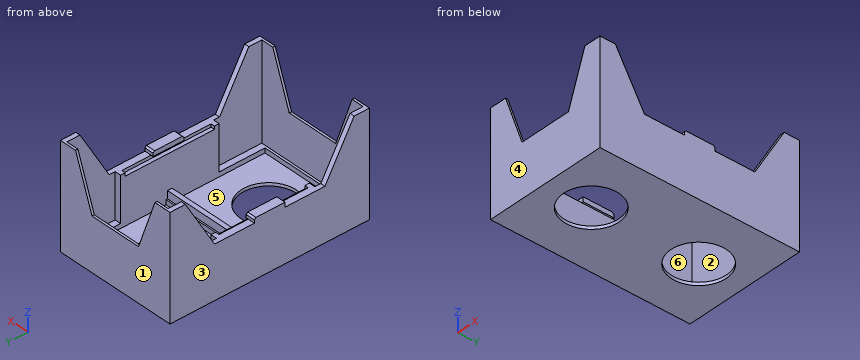
```python
from build123d import *

# Parameters (mm, degrees)
SKETCH1_W                    = 130
SKETCH1_H                    = 80
SKETCH1_R                    = 18
BOSS_EXTRUDE1_DEPTH          = 2
SKETCH2_W                    = 7
SKETCH2_H                    = 130
BOSS_EXTRUDE2_DEPTH          = 30
BOSS_EXTRUDE3_DEPTH          = 35
SKETCH5_W                    = 150
SKETCH5_H                    = 110
CUT_EXTRUDE1_DEPTH           = 33
CUT_EXTRUDE1_DRAFT           = -30
SKETCH6_W                    = 6
SKETCH6_H                    = 20
BOSS_EXTRUDE4_DEPTH          = 3
CHAMFER1_SIZE                = 1
SKETCH7_W                    = 80
SKETCH7_H                    = 5
SKETCH7_H_2                  = 3
BOSS_EXTRUDE5_DEPTH          = 3
SKETCH9_W                    = 74
SKETCH9_H                    = 32.9
CUT_EXTRUDE2_DEPTH           = 99.33107342
SKETCH10_W                   = 72.40522931
SKETCH10_H                   = 3
BOSS_EXTRUDE6_DEPTH          = 5
SKETCH11_W                   = 80
SKETCH11_H                   = 1.5
BOSS_EXTRUDE7_DEPTH          = 62
SKETCH12_W                   = 58
SKETCH12_H                   = 28.83651326
CUT_EXTRUDE3_DEPTH           = 33
CUT_EXTRUDE3_DRAFT           = -20
CUT_EXTRUDE3_PROFILE_2_DEPTH = 33
CUT_EXTRUDE3_PROFILE_2_DRAFT = -20


with BuildPart() as part:
    # Sketch1 → Boss-Extrude1 (new body)
    with BuildSketch(Plane(origin=(0, 0, 0), x_dir=(0, 1, 0), z_dir=(0, 0, 1))):
        Rectangle(SKETCH1_W, SKETCH1_H)
        with Locations(Location((-35, 0, 0), (0, 0, 270))):
            Circle(SKETCH1_R, mode=Mode.SUBTRACT)
        with Locations(Location((35, 0, 0), (0, 0, 90))):
            Circle(SKETCH1_R, mode=Mode.SUBTRACT)
    extrude(amount=BOSS_EXTRUDE1_DEPTH)

    # Sketch2 → Boss-Extrude2 (add)
    with BuildSketch(Plane.XY.offset(2)):
        with Locations((-36.5, 0)):
            Rectangle(SKETCH2_W, SKETCH2_H)
        with Locations((36.5, 0)):
            Rectangle(SKETCH2_W, SKETCH2_H)
    extrude(amount=BOSS_EXTRUDE2_DEPTH)

    # Sketch4 → Boss-Extrude3 (add)
    with BuildSketch(Plane.XY.offset(32)):
        Polygon((-33, 29.1), (-35.5, 29.1), (-35.5, -29.1), (-33, -29.1), (-33, -65), (-40, -65), (-40, 65), (-33, 65), align=None)
        Polygon((35.5, -29.1), (35.5, 29.1), (33, 29.1), (33, 65), (40, 65), (40, -65), (33, -65), (33, -29.1), align=None)
    extrude(amount=BOSS_EXTRUDE3_DEPTH)


with BuildPart() as cut_extrude1_tool:
    # Sketch5 → Cut-Extrude1 (with draft: the straight prism first)
    with BuildSketch(Plane.XY.offset(67)):
        Rectangle(SKETCH5_W, SKETCH5_H)
    extrude(amount=-CUT_EXTRUDE1_DEPTH)
    # Cut-Extrude1: the draft: its side faces are tilted about the plane it starts from
    cut_extrude1_sides = [cut_extrude1_tool.faces().sort_by_distance(p)[0] for p in [
        (0, -55, 50.5),
        (75, 0, 50.5),
        (0, 55, 50.5),
        (-75, 0, 50.5),
    ]]
    draft(cut_extrude1_sides, Plane.XY.offset(67), CUT_EXTRUDE1_DRAFT)


with BuildPart() as part_1:
    add(part.part)

    # Cut-Extrude1: cut by cut_extrude1_tool
    add(cut_extrude1_tool.part, mode=Mode.SUBTRACT)

    # Sketch6 → Boss-Extrude4 (add)
    with BuildSketch(Plane.XY.offset(34)):
        with Locations((37, 0)):
            Rectangle(SKETCH6_W, SKETCH6_H)
        with Locations((-37, 0)):
            Rectangle(SKETCH6_W, SKETCH6_H)
    extrude(amount=BOSS_EXTRUDE4_DEPTH)

    # Chamfer1
    chamfer1_edges = [part_1.edges().sort_by_distance(p)[0] for p in [
        (37, 10, 37),
        (37, -10, 37),
        (-37, 10, 37),
    ]]
    chamfer(chamfer1_edges, length=CHAMFER1_SIZE)

    # Sketch7 → Boss-Extrude5 (add)
    with BuildSketch(Plane.XY.offset(2)):
        Rectangle(SKETCH7_W, SKETCH7_H)
        with Locations((0, -63.5)):
            Rectangle(SKETCH7_W, SKETCH7_H_2)
        with Locations((0, 63.5)):
            Rectangle(SKETCH7_W, SKETCH7_H_2)
    extrude(amount=BOSS_EXTRUDE5_DEPTH)

    # Sketch9 → Cut-Extrude2 (cut, through all)
    with BuildSketch(Plane.XY.offset(5)):
        with Locations((0, 48.55)):
            Rectangle(SKETCH9_W, SKETCH9_H)
        with Locations((0, -48.55)):
            Rectangle(SKETCH9_W, SKETCH9_H)
    extrude(amount=CUT_EXTRUDE2_DEPTH, mode=Mode.SUBTRACT)

    # Sketch10 → Boss-Extrude6 (add)
    with BuildSketch(Plane.XY.offset(5)):
        Rectangle(SKETCH10_W, SKETCH10_H)
    extrude(amount=BOSS_EXTRUDE6_DEPTH)

    # Sketch11 → Boss-Extrude7 (add)
    with BuildSketch(Plane.XY.offset(5)):
        with Locations((0, 64.25)):
            Rectangle(SKETCH11_W, SKETCH11_H)
        with Locations((0, -64.25)):
            Rectangle(SKETCH11_W, SKETCH11_H)
    extrude(amount=BOSS_EXTRUDE7_DEPTH)


with BuildPart() as cut_extrude3_tool:
    # Sketch12 → Cut-Extrude3 (with draft: the straight prism first)
    with BuildSketch(Plane.XY.offset(67)):
        with Locations((0, 63.5)):
            Rectangle(SKETCH12_W, SKETCH12_H)
    extrude(amount=-CUT_EXTRUDE3_DEPTH)
    # Cut-Extrude3: the draft: its side faces are tilted about the plane it starts from
    cut_extrude3_sides = [cut_extrude3_tool.faces().sort_by_distance(p)[0] for p in [
        (0, 49.08174337, 50.5),
        (29, 63.5, 50.5),
        (0, 77.91825663, 50.5),
        (-29, 63.5, 50.5),
    ]]
    draft(cut_extrude3_sides, Plane.XY.offset(67), CUT_EXTRUDE3_DRAFT)


with BuildPart() as part_2:
    add(part_1.part)

    # Cut-Extrude3: cut by cut_extrude3_tool
    add(cut_extrude3_tool.part, mode=Mode.SUBTRACT)


with BuildPart() as cut_extrude3_profile_2_tool:
    # Sketch12 → Cut-Extrude3 profile 2 (with draft: the straight prism first)
    with BuildSketch(Plane.XY.offset(67)):
        with Locations((0, -63.5)):
            Rectangle(SKETCH12_W, SKETCH12_H)
    extrude(amount=-CUT_EXTRUDE3_PROFILE_2_DEPTH)
    # Cut-Extrude3 profile 2: the draft: its side faces are tilted about the plane it starts from
    cut_extrude3_profile_2_sides = [cut_extrude3_profile_2_tool.faces().sort_by_distance(p)[0] for p in [
        (-29, -63.5, 50.5),
        (0, -77.91825663, 50.5),
        (29, -63.5, 50.5),
        (0, -49.08174337, 50.5),
    ]]
    draft(cut_extrude3_profile_2_sides, Plane.XY.offset(67), CUT_EXTRUDE3_PROFILE_2_DRAFT)


with BuildPart() as part_3:
    add(part_2.part)

    # Cut-Extrude3 profile 2: cut by cut_extrude3_profile_2_tool
    add(cut_extrude3_profile_2_tool.part, mode=Mode.SUBTRACT)


solid = part_3.part
```
Geometry: final body of the model. Coordinates: model frame, mm. Face numbers are marked on the shaded views. A direction names the side the tool comes from. Give positions to 0.01 mm unless a question says otherwise; leave off trailing zeros. Loops run counter-clockwise (first coordinate to the right, second up) from the corner with the lowest first, then second, coordinate; pieces in that order, holes last. Notation, with made-up numbers: (-5, 83.5) - (14, 83.5) arc R22 ccw to (14, 122.5) - close; hole circle Ø9 at (60.5, -35). An arc over 180 degrees is marked (long way). Answer as CSV lines item,"result". Start each with the question number.
(1) Section query D-D (y = -56.5). Output: boundary loops of the cut face in (x, z).
(2) Section query B-B (z = 55.5). Output: boundary loops of the cut face in (x, y), and give its area (3 significant figures).
(3) Reachability of the marked faces 1 and 2 from +Z, -Z, +X, -X, +Y, -Y: full face, straight path, thin tool, end or side. Return the list, or none.
(4) Mould query, pull axis X, two halves, no side actions, for the marked faces 3, 4, 5 and 6. Classes: +X half, -X half, draft (parallel to the pull), parting line (faces both ways), or undercut.
(5) Section query A-A (z = 25). Output: boundary loops of the cut face in (x, y).
(6) Ray query, line 1 along Y through (x, z) = (0, 0.55); line 2 along X through (y, z) = (-57, 55); line 3 along X through (y, z) = (-14, 16.5). Return the intervals inside material, ascending. Write a range as [from, to].
(7) Section query C-C (x = 11). Output: boundary loops of the cut face in (y, z).
(8) Pin query (flat end, axial travel): P1, Ø3, axis at x = -34, y = 9.5, coming from the +Z side; P2, Ø0.5, axis at x = -9, y = -2, coming from the +Z side; P3, Ø3.5, axis at x = -35.5, y = -26.5, coming from the +Z side; P4, Ø10, axis at y = 19.5, z = 43, coming from the +X side. Return the tip coordinate at first contact, or that it passes through.
Worked answers:
1,outline,"(-40, 0) - (40, 0) - (40, 67) - (37, 67) - (37, 5) - (33, 5) - (33, 2) - (-33, 2) - (-33, 5) - (-37, 5) - (-37, 67) - (-40, 67) - close"
2,outline,"(-40, -65) - (-24.81, -65) - (-24.81, -63.5) - (-37, -63.5) - (-37, -48.36) - (-40, -48.36) - close; (-40, 48.36) - (-37, 48.36) - (-37, 63.5) - (-24.81, 63.5) - (-24.81, 65) - (-40, 65) - close; (24.81, -65) - (40, -65) - (40, -48.36) - (37, -48.36) - (37, -63.5) - (24.81, -63.5) - close; (24.81, 63.5) - (37, 63.5) - (37, 48.36) - (40, 48.36) - (40, 65) - (24.81, 65) - close"
2,area,"273 mm^2"
3,face 1,"+Z, -Z, +X, -X, +Y"
3,face 2,"+Z"
4,face 3,"-X half"
4,face 4,"draft"
4,face 5,"undercut"
4,face 6,"undercut"
5,outline,"(-40, -65) - (40, -65) - (40, 65) - (-40, 65) - close; hole (-37, -63.5) - (37, -63.5) - (37, -32.1) - (33, -32.1) - (33, 32.1) - (37, 32.1) - (37, 63.5) - (-37, 63.5) - (-37, 32.1) - (-33, 32.1) - (-33, -32.1) - (-37, -32.1) - close"
6,line 1,"y = [-65, -53], [-17, 17], [53, 65]"
6,line 2,"x = [-40, -37], [37, 40]"
6,line 3,"x = [-40, -33], [33, 40]"
7,outline,"(-65, 0) - (-49.25, 0) - (-49.25, 2) - (-62, 2) - (-62, 5) - (-63.5, 5) - (-63.5, 34) - (-65, 34) - close; (-20.75, 0) - (20.75, 0) - (20.75, 2) - (2.5, 2) - (2.5, 5) - (1.5, 5) - (1.5, 10) - (-1.5, 10) - (-1.5, 5) - (-2.5, 5) - (-2.5, 2) - (-20.75, 2) - close; (49.25, 0) - (65, 0) - (65, 34) - (63.5, 34) - (63.5, 5) - (62, 5) - (62, 2) - (49.25, 2) - close"
8,P1,"stops at z = 37"
8,P2,"stops at z = 5"
8,P3,"stops at z = 34"
8,P4,"passes through"
